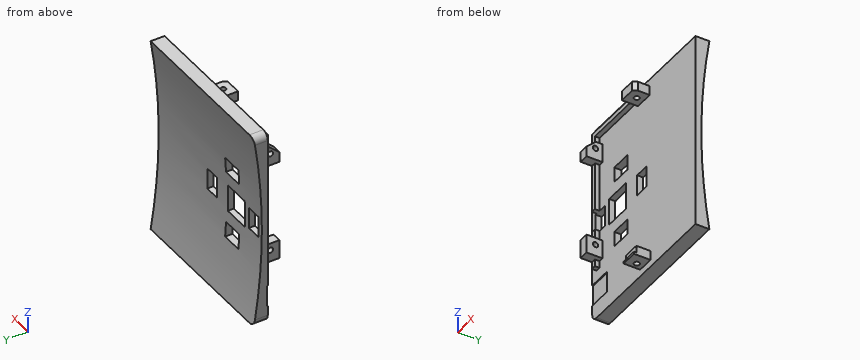
```python
from build123d import *

# Parameters (mm, degrees)
SKETCH009_W             = 84
SKETCH009_H             = 70
PAD002_DEPTH            = 2
SKETCH010_W             = 2
SKETCH010_H             = 7
PAD003_DEPTH            = 2
SKETCH012_W             = 8
SKETCH012_H             = 6.8
PAD004_DEPTH            = 4
SKETCH013_W             = 7
SKETCH013_H             = 6
PAD005_DEPTH            = 4
SKETCH011_W             = 8
SKETCH011_H             = 6.8
PAD006_DEPTH            = 4
SKETCH014_R             = 1.15
POCKET002_DEPTH         = 81.001
SKETCH016_R             = 1.15
POCKET003_DEPTH         = 8.501
SKETCH018_W             = 11.5
SKETCH018_H             = 11.5
POCKET004_DEPTH         = 5
POCKET005_DEPTH         = 5
POCKET006_DEPTH         = 5
SKETCH021_W             = 1
SKETCH021_H             = 7
PAD007_DEPTH            = 1
SKETCH022_W             = 9
SKETCH022_H             = 10
POCKET007_DEPTH         = 0.4
FILLET_R                = 3
BODY002_PITCH_ANGLE     = -90
BODY002_PLACEMENT_ANGLE = 90
PAD001_DEPTH            = 35
SKETCH007_W             = 11.5
SKETCH007_H             = 11.5
POCKET001_DEPTH         = 13
FILLET001_R             = 3
SKETCH025_W             = 6.5
SKETCH025_H             = 9
SKETCH025_W_2           = 9
SKETCH025_H_2           = 6.5
POCKET008_DEPTH         = 8


with BuildPart() as back:
    # Sketch009 → Pad002 (new body)
    with BuildSketch(Plane.XY):
        Rectangle(SKETCH009_W, SKETCH009_H)
    extrude(amount=PAD002_DEPTH)

    # Sketch010 (on Face6 of Pad002) → Pad003 (join)
    with BuildSketch(Plane.XY.offset(2)):
        with Locations((-38, -1)):
            Rectangle(SKETCH010_W, SKETCH010_H)
        Polygon((-21, 32), (39, 32), (39, -4), (37, -4), (37, 30), (-21, 30), align=None)
    extrude(amount=PAD003_DEPTH)

    # Sketch012 (on Face15 of Pad003) → Pad004 (join)
    with BuildSketch(Plane.YZ.offset(39)):
        with Locations((0, 5.4)):
            Rectangle(SKETCH012_W, SKETCH012_H)
    extrude(amount=-PAD004_DEPTH)

    # Sketch013 (on Face9 of Pad004) → Pad005 (join)
    with BuildSketch(Plane(origin=(-39, 0, 0), x_dir=(0, -1, 0), z_dir=(-1, 0, 0))):
        with Locations((1, 5)):
            Rectangle(SKETCH013_W, SKETCH013_H)
    extrude(amount=-PAD005_DEPTH)

    # Sketch011 (on Face16 of Pad003) → Pad006 (join)
    with BuildSketch(Plane(origin=(0, 32, 0), x_dir=(-1, 0, 0), z_dir=(0, 1, 0))):
        with Locations((-29, 5.4)):
            Rectangle(SKETCH011_W, SKETCH011_H)
        with Locations((14, 5.4)):
            Rectangle(SKETCH011_W, SKETCH011_H)
    extrude(amount=-PAD006_DEPTH)

    # Sketch014 (on Face44 of Pad006) → Pocket002 (cut, through all)
    with BuildSketch(Plane.YZ.offset(39)):
        with Locations((0, 5)):
            Circle(SKETCH014_R)
    extrude(amount=-POCKET002_DEPTH, mode=Mode.SUBTRACT)

    # Sketch016 → Pocket003 (cut, through all)
    with BuildSketch(Plane.XZ.offset(-26.5)):
        with Locations((-13, 5)):
            Circle(SKETCH016_R)
        with Locations((30, 5)):
            Circle(SKETCH016_R)
    extrude(amount=-POCKET003_DEPTH, mode=Mode.SUBTRACT)

    # Sketch018 (on Face5 of Pocket003) → Pocket004 (cut)
    with BuildSketch(Plane.XY.offset(2)):
        with Locations((0, 17.75)):
            Rectangle(SKETCH018_W, SKETCH018_H)
    extrude(amount=-POCKET004_DEPTH, mode=Mode.SUBTRACT)

    # Sketch019 (on Face31 of Pocket004) → Pocket005 (cut)
    with BuildSketch(Plane.XZ.offset(-28)):
        Polygon((29.125944, 9.042901), (33.258869, 4.499726), (33.258869, 9.042901), align=None)
    extrude(amount=-POCKET005_DEPTH, mode=Mode.SUBTRACT)

    # Sketch020 (on Face36 of Pocket005) → Pocket006 (cut)
    with BuildSketch(Plane(origin=(35, 0, 0), x_dir=(0, -1, 0), z_dir=(-1, 0, 0))):
        Polygon((2.77547, 8.938441), (6.386171, 3.079567), (6.386171, 8.938441), align=None)
    extrude(amount=-POCKET006_DEPTH, mode=Mode.SUBTRACT)

    # Sketch021 (on Face40 of Pocket006) → Pad007 (join)
    with BuildSketch(Plane.XY.offset(8)):
        with Locations((-38.5, -1)):
            Rectangle(SKETCH021_W, SKETCH021_H)
    extrude(amount=PAD007_DEPTH)

    # Sketch022 (on Face5 of Pocket005) → Pocket007 (cut)
    with BuildSketch(Plane.XY.offset(2)):
        with Locations((-30.3, 30)):
            Rectangle(SKETCH022_W, SKETCH022_H)
    extrude(amount=-POCKET007_DEPTH, mode=Mode.SUBTRACT)

    # Fillet
    fillet_edges = [back.edges().sort_by_distance(p)[0] for p in [
        (42, 35, 1),
        (-42, 35, 1),
    ]]
    fillet(fillet_edges, radius=FILLET_R)


with BuildPart() as back_1:
    # Body002 pitch: moved
    add(back.part.rotate(Axis((0, 0, 0), (0, 1, 0)), BODY002_PITCH_ANGLE))


with BuildPart() as back_2:
    # Body002 placement: moved
    add(back_1.part.rotate(Axis((0, 0, 0), (0, 0, 1)), BODY002_PLACEMENT_ANGLE))


with BuildPart() as curve:
    # Sketch006 → Pad001 (new body, symmetric)
    with BuildSketch(Plane(origin=(0, 0, 0), x_dir=(0, 0, -1), z_dir=(1, 0, 0))):
        with BuildLine():
            ThreePointArc((-42, 3.9), (0, 0.511678), (42, 3.9))
            Line((42, -0.1), (42, 3.9))
            Line((-42, -0.1), (42, -0.1))
            Line((-42, 3.9), (-42, -0.1))
        make_face()
    extrude(amount=PAD001_DEPTH, both=True)

    # Sketch007 (on Face3 of Pad001) → Pocket001 (cut)
    with BuildSketch(Plane.XZ.offset(0.1)):
        with Locations((-17.75, 0)):
            Rectangle(SKETCH007_W, SKETCH007_H)
    extrude(amount=-POCKET001_DEPTH, mode=Mode.SUBTRACT)

    # Fillet001
    fillet001_edges = [curve.edges().sort_by_distance(p)[0] for p in [
        (-35, 1.9, -42),
        (-35, 1.9, 42),
    ]]
    fillet(fillet001_edges, radius=FILLET001_R)

    # Boolean: union Back
    add(back_2.part)

    # Sketch025 (on Face32 of Boolean) → Pocket008 (cut, symmetric)
    with BuildSketch(Plane.XZ.offset(2)):
        with Locations((-29.5, 0)):
            Rectangle(SKETCH025_W, SKETCH025_H)
        with Locations((-15.55, 14.375)):
            Rectangle(SKETCH025_W_2, SKETCH025_H_2)
        with Locations((-1.3, 0)):
            Rectangle(SKETCH025_W, SKETCH025_H)
        with Locations((-15.55, -14.375)):
            Rectangle(SKETCH025_W_2, SKETCH025_H_2)
    extrude(amount=POCKET008_DEPTH, both=True, mode=Mode.SUBTRACT)


solid = curve.part
```
The listing builds one solid part. Answer for the finished solid, in the listing's coordinates (mm). Give positions to 0.01 mm unless a question says otherwise; leave off trailing zeros. Order: outer loops, then holes, each group sorted by start corner. A loop starts at its lowest first (then second) coordinate and runs counter-clockwise, first axis right, second up. Notation, with made-up numbers: (-5, 69) -> (48, 69) arc R10 cw to (48, 76) -> close; hole circle Ø8 at (15.5, 56.5). An arc over 180 degrees is marked (long way). One line per item, written item: value.
1) Find section B-B, the plane z = -13. Determine the outline of the cut face in (x, y), plus the area to 3 significant figures.
Reported:
outline: (-35, -2) -> (-32, -2) -> (-32, -3.85) -> (-28, -3.85) -> (-28, -2) -> (-20.05, -2) -> (-20.05, 0.83) -> (-35, 0.83) -> close; (-32, -8.8) -> (-28, -8.8) -> (-28, -6.15) -> (-32, -6.15) -> close; (-11.05, -2) -> (35, -2) -> (35, 0.83) -> (-11.05, 0.83) -> close
area: 191 mm^2
2) Flat-ended cylindrical pins translate along their axes: P1, Ø2, axis at y = -5, z = -13, coming from the +X side; P2, Ø12, axis at x = -25, z = 4.5, coming from the -Y side; P3, Ø12, axis at x = 9.5, z = -33.5, coming from the +Y side; P4, Ø4, axis at x = -26, z = -19.5, coming from the +Y side. Find the tip coordinate at first contact, or state that the pin passes through.
Reported:
P1: passes through
P2: stops at y = -4
P3: stops at y = 3.51
P4: stops at y = 1.4
3) Find section C-C, the plane x = 8.5. Determine the outline of the cut face in (y, z), plus the area to 3 significant figures.
Reported:
outline: (-2, -42) -> (3.9, -42) arc R262 cw to (3.9, 42) -> (-2, 42) -> close
area: 306 mm^2
4) Find the intervals of material crossed by line 1 (Z direction, x = -27.5, y = -0.25); line 2 (X direction, y = -5, z = -36.7); line 3 (Z direction, x = -27, y = -3.75), in increasing order.
Reported:
line 1: z = -42 to -4.5, 4.5 to 42
line 2: x = -2.5 to -1.15, 1.15 to 4.5
line 3: z = 37 to 39
5) Find section D-D, the plane z = 8. Determine the outline of the cut face in (x, y).
Reported:
outline: (-35, -2) -> (-32, -2) -> (-32, -4) -> (-30, -4) -> (-30, -2) -> (35, -2) -> (35, 0.63) -> (-35, 0.63) -> close
6) Find section A-A, the plane x = 0. Determine the outline of the cut face in (y, z).
Reported:
outline: (-9, -39) -> (-6.15, -39) -> (-6.15, -35) -> (-8, -35) -> (-8, -38) -> (-9, -38) -> close; (-8.8, 35) -> (-6.15, 35) -> (-6.15, 39) -> (-8.8, 39) -> close; (-3.85, -39) -> (-2, -39) -> (-2, -42) -> (3.9, -42) arc R262 cw to (0.55, -4.5) -> (-2, -4.5) -> (-2, -35) -> (-3.85, -35) -> close; (-3.85, 35) -> (-2, 35) -> (-2, 4.5) -> (0.55, 4.5) arc R262 cw to (3.9, 42) -> (-2, 42) -> (-2, 39) -> (-3.85, 39) -> close
